```python
from build123d import *

# Parameters (mm, degrees)
BOSS_EXTRUDE1_DEPTH = 70
SKETCH2_R           = 1.5
CUT_EXTRUDE1_DEPTH  = 70


with BuildPart() as part:
    # Sketch1 → Boss-Extrude1 (new body)
    with BuildSketch(Plane.XY):
        Polygon((0, 0), (0, 55), (3, 55), (3, 3), (70, 3), (70, 0), align=None)
    extrude(amount=BOSS_EXTRUDE1_DEPTH)

    # Sketch2 → Cut-Extrude1 (cut)
    with BuildSketch(Plane(origin=(3, 0, 0), x_dir=(0, 0, -1), z_dir=(1, 0, 0))):
        with Locations((-50, 43)):
            Circle(SKETCH2_R)
        with Locations((-20, 43)):
            Circle(SKETCH2_R)
        with Locations((-20, 15)):
            Circle(SKETCH2_R)
        with Locations((-50, 15)):
            Circle(SKETCH2_R)
    extrude(amount=-CUT_EXTRUDE1_DEPTH, mode=Mode.SUBTRACT)


solid = part.part
```
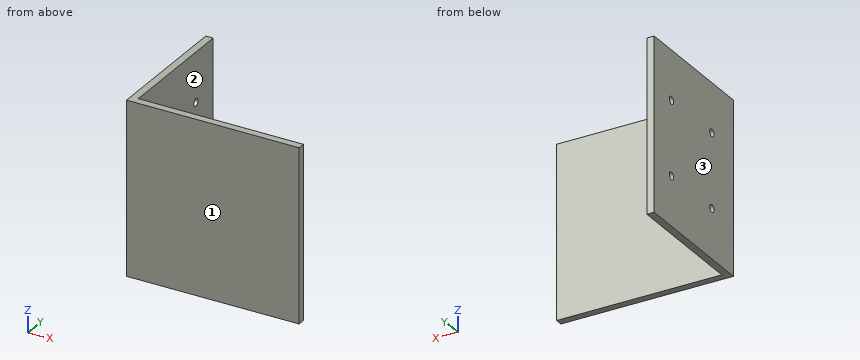
Design review of the part built by this model. Coordinates are the model's own, in mm. Face numbers are marked on the shaded views. Coordinates: 2 decimals unless noted, no trailing zeros. Order: outer loops, then holes, each group sorted by start corner. A loop starts at its lowest first (then second) coordinate and runs counter-clockwise, first axis right, second up.
1) Take a section at C-C, the plane z = 7. Give the boundary of the cut face in (x, y), and give its area (3 significant figures).
2) Clearance check with flat-ended pins moving along their axes: pin 1 (20 mm diameter, centred on x = 26, z = 48, fed in from +Y); pin 2 (3 mm diameter, centred on y = 39, z = 11, fed in from +X). State where each tip first meets the part, or that it passes through.
3) Wall thickness on line 1 along Y through (x, z) = (2, 20); line 2 along X through (y, z) = (32, 15.5): over which ranges is each line inside the solid? List them lowest first.
4) Mouldability with a two-part tool opening along X and no side actions: class the marked faces 1, 2 and 3 as +X half, -X half, draft (parallel to the pull), parting line (faces both ways), or undercut.
5) Take a section at D-D, the plane x = 38. Give the boundary of the cut face in (y, z).
6) Take a section at A-A, the plane y = 15. Give the boundary of the cut face in (x, z).
7) Take a section at B-B, the plane z = 50. Give the boundary of the cut face in (x, y), and give its area (3 significant figures).
Returned:
1. outline: (0, 0) - (70, 0) - (70, 3) - (3, 3) - (3, 55) - (0, 55) - close
1. area: 366 mm2
2. pin 1: stops at y = 3
2. pin 2: stops at x = 3
3. line 1: y = 0 to 13.5, 16.5 to 41.5, 44.5 to 55
3. line 2: x = 0 to 3
4. face 1: draft
4. face 2: +X half
4. face 3: -X half
5. outline: (0, 0) - (3, 0) - (3, 70) - (0, 70) - close
6. outline: (0, 0) - (3, 0) - (3, 18.5) - (0, 18.5) - close; (0, 21.5) - (3, 21.5) - (3, 48.5) - (0, 48.5) - close; (0, 51.5) - (3, 51.5) - (3, 70) - (0, 70) - close
7. outline: (0, 0) - (70, 0) - (70, 3) - (3, 3) - (3, 13.5) - (0, 13.5) - close; (0, 16.5) - (3, 16.5) - (3, 41.5) - (0, 41.5) - close; (0, 44.5) - (3, 44.5) - (3, 55) - (0, 55) - close
7. area: 348 mm2
